Input: dimensioned drawing with shaded views. Units: mm. Origin: part minimum x, y, z. A direction names the side the tool comes from. Round coordinates to 2 decimals unless told otherwise and drop trailing zeros. Loops run counter-clockwise (first coordinate to the right, second up) from the corner with the lowest first, then second, coordinate; pieces in that order, holes last. Notation, with made-up numbers: (-8, 67.25) - (30, 67.25) arc R25 ccw to (30, 83.25) - close; hole circle Ø8 at (18, 15). An arc over 180 degrees is marked (long way). One line per question, with ' | ' between items. Start each with the question number.
Item 1: Section D-D, the plane x = 35.5. Return loops of the section in (y, z).
Item 2: Set-up query: the marked faces 5, 6, 7 and 8. Return all of +Z, -Z, +X, -X, +Y, -Y with unobstructed straight access to the full face (end or side cutting, diameter ignored); none if empty.
Item 3: Section B-B, the plane x = 3.5. Return loops of the section in (y, z), plus the area to 4 significant figures.
Item 4: Section C-C, the plane y = 10.25. Return loops of the section in (x, z).
Item 5: Draft query along X for the marked faces 1, 2, 3 and 4. Return one class per face: pulls with the +X half, pulls with the -X half, needs draft (parallel to the pull), parting line crosses it, or undercut.
Item 6: First-contact query: pin 1 (1.5 mm diameter, centred on y = 19, z = 2, fed in from +X); pin 2 (13 mm diameter, centred on x = 4, z = 23, fed in from +Y); pin 3 (6 mm diameter, centred on x = 26.5, y = 11, fed in from -Z). Flat tips, straight axial feed; report the tip coordinate or a pass-through.
Item 7: Section A-A, the plane z = 34.6. Return loops of the section in (x, y), plus the area to 3 significant figures.
Item 8: Material intervals for line 1 along Z through (x, y) = (3.5, 2.3); line 2 along Y through (x, z) = (8, 1); line 3 along Z through (x, y) = (20.5, 8.5), sorted ascending.
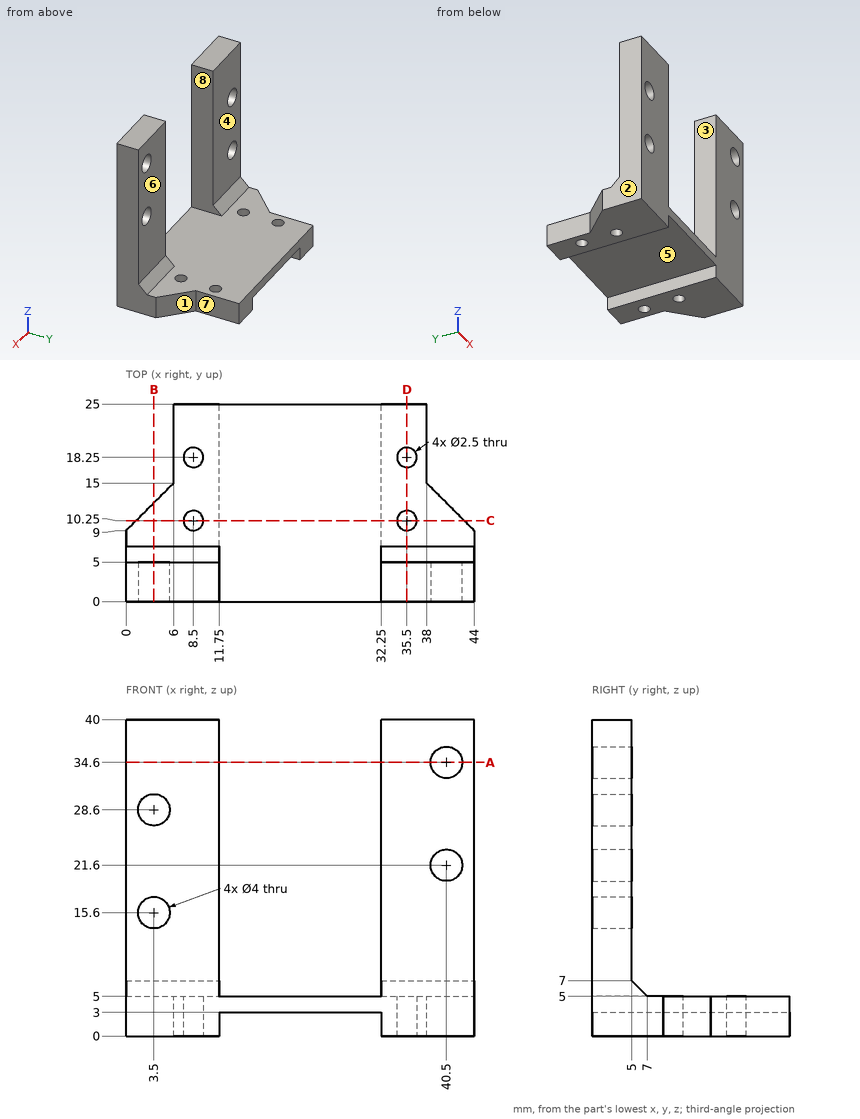
Return value:
1) outline: (0, 0) - (9, 0) - (9, 5) - (7, 5) - (5, 7) - (5, 40) - (0, 40) - close; (11.5, 0) - (17, 0) - (17, 5) - (11.5, 5) - close; (19.5, 0) - (25, 0) - (25, 5) - (19.5, 5) - close
2) face 5: -Z, +Y, -Y | face 6: +Z, +X, -X, +Y | face 7: +Z, -Z, +X, +Y | face 8: +Z, +Y, -Y
3) outline: (0, 0) - (12.5, 0) - (12.5, 5) - (7, 5) - (5, 7) - (5, 13.6) - (0, 13.6) - close; (0, 17.6) - (5, 17.6) - (5, 26.6) - (0, 26.6) - close; (0, 30.6) - (5, 30.6) - (5, 40) - (0, 40) - close | area: 199.5 mm2
4) outline: (1.25, 0) - (7.25, 0) - (7.25, 5) - (1.25, 5) - close; (9.75, 0) - (11.75, 0) - (11.75, 3) - (32.25, 3) - (32.25, 0) - (34.25, 0) - (34.25, 5) - (9.75, 5) - close; (36.75, 0) - (42.75, 0) - (42.75, 5) - (36.75, 5) - close
5) face 1: pulls with the +X half | face 2: pulls with the -X half | face 3: undercut | face 4: needs draft
6) pin 1: x = 38 | pin 2: y = 5 | pin 3: z = 3
7) outline: (0, 0) - (11.75, 0) - (11.75, 5) - (0, 5) - close; (32.25, 0) - (38.5, 0) - (38.5, 5) - (32.25, 5) - close; (42.5, 0) - (44, 0) - (44, 5) - (42.5, 5) - close | area: 97.5 mm2
8) line 1: 0 to 13.6, 17.6 to 26.6, 30.6 to 40 | line 2: 0 to 9.1, 11.4 to 17.1, 19.4 to 25 | line 3: 3 to 5
